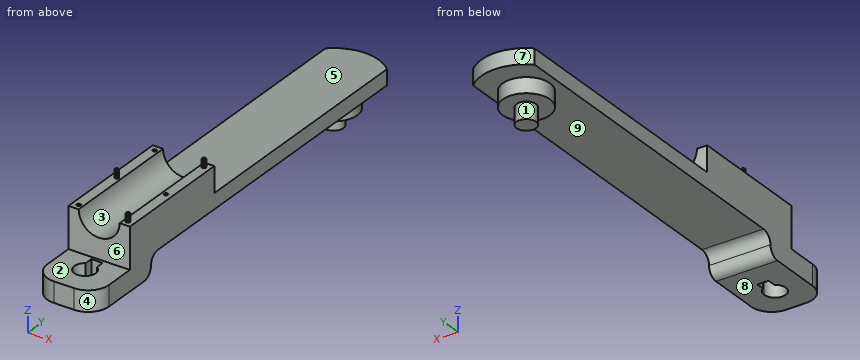
```python
from build123d import *

# Parameters (mm, degrees)
SKETCH2_W                  = 30
SKETCH2_H                  = 30
BOSS_EXTRUDE1_DEPTH        = 60
FILLET1_R                  = 10
SKETCH3_W                  = 40
SKETCH3_H                  = 25
CUT_EXTRUDE1_DEPTH         = 69.738635424
SKETCH6_W                  = 30
SKETCH6_H                  = 40
BOSS_EXTRUDE2_DEPTH        = 125
SKETCH7_W                  = 30
SKETCH7_H                  = 10
BOSS_EXTRUDE3_DEPTH        = 10
FILLET2_START              = -16
FILLET2_DEPTH              = 32
FILLET2_START_2            = -15
FILLET2_2_DEPTH            = 30
SKETCH8_W                  = 25
SKETCH8_H                  = 70
CUT_EXTRUDE2_DEPTH         = 156.241746963
SKETCH12_W                 = 30
SKETCH12_H                 = 7.5
BOSS_EXTRUDE4_DEPTH        = 65
SKETCH13_W                 = 20
SKETCH13_H                 = 54
CUT_EXTRUDE6_DEPTH         = 6
SKETCH20_R                 = 4.75
AXIS_BASE_DEPTH            = 49.6
CUT_EXTRUDE8_DEPTH         = 212.541958013
CUT_EXTRUDE8_DEPTH_BACK    = 212.541958013
SKETCH19_R                 = 2.5
SKETCH19_W                 = 20
SKETCH19_H                 = 42
CUT_EXTRUDE7_DEPTH         = 26.5
MAKE_HALF_DEPTH            = 225.175347112
ONE_MALE_JACK_DEPTH        = 4
CHAMFER1_SIZE              = 0.2
LPATTERN1_COUNT            = 2
LPATTERN1_PITCH            = 24
LPATTERN1_COUNT_DIR2       = 3
LPATTERN1_PITCH_DIR2       = 27
CHAMFER1_OF_LPATTERN1_SIZE = 0.2
ONE_FEMALE_JACK_DEPTH      = 5
FEMALE_JACKS_COUNT         = 2
FEMALE_JACKS_PITCH         = 24
FEMALE_JACKS_COUNT_DIR2    = 3
FEMALE_JACKS_PITCH_DIR2    = 27
SKETCH26_R                 = 10
MAKE_LIGHER_DEPTH          = 60
SKETCH27_R                 = 11.517379081
BOSS_EXTRUDE5_DEPTH        = 7.45


with BuildPart() as part:
    # Sketch2 → Boss-Extrude1 (new body)
    with BuildSketch(Plane.XY):
        Rectangle(SKETCH2_W, SKETCH2_H)
        with BuildLine():
            ThreePointArc((5.25, 0), (-2.561737691, -4.582575695), (-2.75, 4.472135955))
            Line((-2.75, 4.472135955), (-2.75, 8.5))
            Line((-2.75, 8.5), (0, 8.5))
            Line((0, 8.5), (2.75, 8.5))
            Line((2.75, 8.5), (2.75, 4.472135955))
            ThreePointArc((2.75, 4.472135955), (4.582575695, 2.561737691), (5.25, 0))
        make_face(mode=Mode.SUBTRACT)
    extrude(amount=BOSS_EXTRUDE1_DEPTH)

    # Fillet1
    fillet1_edges = [part.edges().sort_by_distance(p)[0] for p in [
        (15, -15, 30),
        (-15, -15, 30),
    ]]
    fillet(fillet1_edges, radius=FILLET1_R)

    # Sketch3 → Cut-Extrude1 (cut, through all)
    with BuildSketch(Plane.ZY.offset(15)):
        with Locations((30, -2.5)):
            Rectangle(SKETCH3_W, SKETCH3_H)
    extrude(amount=-CUT_EXTRUDE1_DEPTH, mode=Mode.SUBTRACT)

    # Sketch6 → Boss-Extrude2 (add)
    with BuildSketch(Plane(origin=(0, 15, 0), x_dir=(1, 0, 0), z_dir=(0, 1, 0))):
        with Locations((0, -30)):
            Rectangle(SKETCH6_W, SKETCH6_H)
    extrude(amount=BOSS_EXTRUDE2_DEPTH)

    # Sketch7 → Boss-Extrude3 (add)
    with BuildSketch(Plane(origin=(0, 15, 0), x_dir=(1, 0, 0), z_dir=(0, 1, 0))):
        with Locations((0, -5)):
            Rectangle(SKETCH7_W, SKETCH7_H)
        with Locations((0, -55)):
            Rectangle(SKETCH7_W, SKETCH7_H)
    extrude(amount=BOSS_EXTRUDE3_DEPTH)

    # Fillet2: read off the stored shape, not the designer's step
    # Fillet2 outline → Fillet2 (cut)
    with BuildSketch(Plane.YZ.offset(FILLET2_START)):
        with BuildLine():
            ThreePointArc((25, 5), (23.535533906, 1.464466094), (20, 0))
            Line((20, 0), (25, 0))
            Line((25, 0), (25, 5))
        make_face()
        with BuildLine():
            Line((25, 60), (20, 60))
            ThreePointArc((20, 60), (23.535533906, 58.535533906), (25, 55))
            Line((25, 55), (25, 60))
        make_face()
    extrude(amount=FILLET2_DEPTH, mode=Mode.SUBTRACT)

    # Fillet2 2 outline → Fillet2 2 (add)
    with BuildSketch(Plane.YZ.offset(FILLET2_START_2)):
        with BuildLine():
            Line((25, 10), (25, 5))
            ThreePointArc((25, 5), (26.464466094, 8.535533906), (30, 10))
            Line((30, 10), (25, 10))
        make_face()
        with BuildLine():
            ThreePointArc((30, 50), (26.464466094, 51.464466094), (25, 55))
            Line((25, 55), (25, 50))
            Line((25, 50), (30, 50))
        make_face()
    extrude(amount=FILLET2_2_DEPTH)

    # Sketch8 → Cut-Extrude2 (cut, through all)
    with BuildSketch(Plane(origin=(15, 0, 0), x_dir=(0, 0, -1), z_dir=(1, 0, 0))):
        with Locations((-30, 105)):
            Rectangle(SKETCH8_W, SKETCH8_H)
    extrude(amount=-CUT_EXTRUDE2_DEPTH, mode=Mode.SUBTRACT)

    # Sketch12 → Boss-Extrude4 (add)
    with BuildSketch(Plane(origin=(0, 140, 0), x_dir=(1, 0, 0), z_dir=(0, 1, 0))):
        with Locations((0, -13.75)):
            Rectangle(SKETCH12_W, SKETCH12_H)
        with Locations((0, -46.25)):
            Rectangle(SKETCH12_W, SKETCH12_H)
    extrude(amount=BOSS_EXTRUDE4_DEPTH)

    # Sketch13 → Cut-Extrude6 (cut)
    with BuildSketch(Plane.XY.offset(50)):
        with Locations((0, 168)):
            Rectangle(SKETCH13_W, SKETCH13_H)
    extrude(amount=-CUT_EXTRUDE6_DEPTH, mode=Mode.SUBTRACT)

    # Sketch20 → Axis Base (add)
    with BuildSketch(Plane.XY.offset(44)):
        with Locations(Location((0, 176.7, 0), (0, 0, 90))):
            Circle(SKETCH20_R)
    extrude(amount=-AXIS_BASE_DEPTH)

    # Sketch23 → Cut-Extrude8 (cut, two sides: drawn at the far end of the back side and taken through both)
    with BuildSketch(Plane(origin=(0, 0, 10), x_dir=(-1, 0, 0), z_dir=(0, 0, -1)).offset(-CUT_EXTRUDE8_DEPTH_BACK)):
        with BuildLine():
            Line((-15, 192.793476939), (-15, 205))
            Line((-15, 205), (15, 205))
            Line((15, 205), (15, 192.793476939))
            ThreePointArc((15, 192.793476939), (0, 198.7), (-15, 192.793476939))
        make_face()
    extrude(amount=CUT_EXTRUDE8_DEPTH + CUT_EXTRUDE8_DEPTH_BACK, mode=Mode.SUBTRACT)

    # Sketch19 → Cut-Extrude7 (cut)
    with BuildSketch(Plane.XY.offset(44)):
        with Locations((-5.12, 192)):
            Circle(SKETCH19_R)
        with Locations(Location((5.12, 192, 0), (0, 0, 270))):
            Circle(SKETCH19_R)
        with Locations((5.12, 144)):
            Circle(SKETCH19_R)
        with Locations(Location((-5.12, 144, 0), (0, 0, 270))):
            Circle(SKETCH19_R)
        with Locations((0, 168)):
            Rectangle(SKETCH19_W, SKETCH19_H)
    extrude(amount=-CUT_EXTRUDE7_DEPTH, mode=Mode.SUBTRACT)

    # 3DSketch2 → Make Half (cut, through all)
    with BuildSketch(Plane(origin=(-16.97773478, -20.308334844, 30), x_dir=(0.14055892995616934, 0.9900723141314359, 0), z_dir=(0, 0, 1))):
        Polygon((0, 0), (4.55547701, -32.087976668), (230.577525736, 0), (226.022048726, 32.087976668), align=None)
    extrude(amount=MAKE_HALF_DEPTH, mode=Mode.SUBTRACT)

    # Sketch24 → One Male Jack (add)
    with BuildSketch(Plane.XY.offset(30)):
        Polygon((12, 68), (11.292893219, 67.707106781), (11, 67), (11.292893219, 66.292893219), (12, 66), (12.707106781, 66.292893219), (13, 67), (12.707106781, 67.707106781), align=None)
    one_male_jack = extrude(amount=ONE_MALE_JACK_DEPTH)

    # Chamfer1
    chamfer1_edges = [part.edges().sort_by_distance(p)[0] for p in [
        (12.353553391, 67.853553391, 34),
        (11.646446609, 67.853553391, 34),
        (11.146446609, 67.353553391, 34),
        (11.146446609, 66.646446609, 34),
        (11.646446609, 66.146446609, 34),
        (12.353553391, 66.146446609, 34),
        (12.853553391, 66.646446609, 34),
        (12.853553391, 67.353553391, 34),
    ]]
    chamfer(chamfer1_edges, length=CHAMFER1_SIZE)

    # LPattern1: One Male Jack 2 × 3, 3 skipped
    with Locations(*[(-i * LPATTERN1_PITCH, -j * LPATTERN1_PITCH_DIR2, 0) for i in range(LPATTERN1_COUNT) for j in range(LPATTERN1_COUNT_DIR2) if (i, j) not in ((0, 0), (0, 1), (1, 0), (1, 2))]):
        add(one_male_jack)

    # Chamfer1 of LPattern1
    chamfer1_of_lpattern1_edges = [part.edges().sort_by_distance(p)[0] for p in [
        (12.353553391, 13.853553391, 34),
        (11.646446609, 13.853553391, 34),
        (11.146446609, 13.353553391, 34),
        (11.146446609, 12.646446609, 34),
        (11.646446609, 12.146446609, 34),
        (12.353553391, 12.146446609, 34),
        (12.853553391, 12.646446609, 34),
        (12.853553391, 13.353553391, 34),
        (-11.646446609, 40.853553391, 34),
        (-12.353553391, 40.853553391, 34),
        (-12.853553391, 40.353553391, 34),
        (-12.853553391, 39.646446609, 34),
        (-12.353553391, 39.146446609, 34),
        (-11.646446609, 39.146446609, 34),
        (-11.146446609, 39.646446609, 34),
        (-11.146446609, 40.353553391, 34),
    ]]
    chamfer(chamfer1_of_lpattern1_edges, length=CHAMFER1_OF_LPATTERN1_SIZE)

    # Sketch25 → One Female Jack (cut)
    with BuildSketch(Plane.XY.offset(30)):
        Polygon((-12, 68.025), (-12.724784451, 67.724784451), (-13.025, 67), (-12.724784451, 66.275215549), (-12, 65.975), (-11.275215549, 66.275215549), (-10.975, 67), (-11.275215549, 67.724784451), align=None)
    one_female_jack = extrude(amount=-ONE_FEMALE_JACK_DEPTH, mode=Mode.SUBTRACT)

    # Female Jacks: One Female Jack 2 × 3, 3 skipped
    with Locations(*[(i * FEMALE_JACKS_PITCH, -j * FEMALE_JACKS_PITCH_DIR2, 0) for i in range(FEMALE_JACKS_COUNT) for j in range(FEMALE_JACKS_COUNT_DIR2) if (i, j) not in ((0, 0), (0, 1), (1, 0), (1, 2))]):
        add(one_female_jack, mode=Mode.SUBTRACT)

    # Sketch26 → Make Ligher (cut)
    with BuildSketch(Plane.XZ.offset(-10)):
        with Locations((0, 30)):
            Circle(SKETCH26_R)
    extrude(amount=-MAKE_LIGHER_DEPTH, mode=Mode.SUBTRACT)

    # Sketch27 → Boss-Extrude5 (add)
    with BuildSketch(Plane(origin=(0, 0, 10), x_dir=(-1, 0, 0), z_dir=(0, 0, -1))):
        with Locations(Location((0, 176.7, 0), (0, 0, 180))):
            Circle(SKETCH27_R)
    extrude(amount=BOSS_EXTRUDE5_DEPTH)


solid = part.part
```
The listing builds one solid part. Answer for the finished solid, in the listing's coordinates (mm). Face numbers are marked on the shaded views. A direction names the side the tool comes from. Give positions to 0.01 mm unless a question says otherwise; leave off trailing zeros. Order: outer loops, then holes, each group sorted by start corner. A loop starts at its lowest first (then second) coordinate and runs counter-clockwise, first axis right, second up. Notation, with made-up numbers: (-14, 21) -> (4, 21) arc R15 cw to (4, 50) -> close; hole circle Ø7 at (10.25, 87). An arc over 180 degrees is marked (long way). Answer as a JSON object with one key per item and string values. Group by question number.
Item 1: The part is cut by section A-A on x = 0. Write down the section's boundary in (y, z).
Item 2: The part is cut by section D-D on y = 48.5. Write down the section's boundary in (x, z), and give its area (3 significant figures).
Item 3: Determine the mould class of the marked faces 6, 7, 8 and 9 for opening direction Y: pulls with the +Y half, pulls with the -Y half, needs draft (parallel to the pull), parting line crosses it, or undercut.
Item 4: The part is cut by section B-B on y = 176.7. Write down the section's boundary in (x, z).
Item 5: The part is cut by section C-C on z = 7. Write down the section's boundary in (x, y), and give its area (3 significant figures).
Item 6: A tool of negligible diameter and unlimited length cuts with its end or side. For the marked faces 1, 2, 3, 4 and 5, from which of +Z, -Z, +X, -X, +Y, -Y can it reach the whole face along a straight path? Write none if from no direction.
Item 7: Flat-ended cylindrical pins translate along their axes: pin 1 (6 mm diameter, centred on x = 6, z = 23.5, fed in from -Y); pin 2 (7 mm diameter, centred on x = 0, y = 181.5, fed in from -Z); pin 3 (4 mm diameter, centred on x = 11.5, y = 46, fed in from +Z); pin 4 (10 mm diameter, centred on x = -12, y = 144, fed in from +Z). Find the tip coordinate at first contact, or state that the pin passes through.
Item 8: Consider L1, parallel to Y at x = 0, z = 4.5; L2, parallel to Y at x = 3, z = 7.5; L3, parallel to X at y = 0, z = 5. Determine where each line is inside the solid, lowest interval first. Write a range as from..to.
Result set:
{
 "1": {"outline": "(-15, 0) -> (-5.25, 0) -> (-5.25, 10) -> (-15, 10) -> close; (8.5, 0) -> (20, 0) arc R5 ccw to (25, 5) arc R5 cw to (30, 10) -> (165.18, 10) -> (165.18, 2.55) -> (171.95, 2.55) -> (171.95, -5.6) -> (181.45, -5.6) -> (181.45, 2.55) -> (188.22, 2.55) -> (188.22, 10) -> (198.7, 10) -> (198.7, 17.5) -> (70, 17.5) -> (70, 20) -> (10, 20) -> (10, 10) -> (8.5, 10) -> close"},
 "2": {"outline": "(-15, 10) -> (15, 10) -> (15, 30) -> (10, 30) arc R10 cw to (-10, 30) -> (-15, 30) -> close", "area": "443 mm²"},
 "3": {"face 6": "pulls with the -Y half", "face 7": "pulls with the +Y half", "face 8": "needs draft", "face 9": "undercut"},
 "4": {"outline": "(-15, 10) -> (-11.52, 10) -> (-11.52, 2.55) -> (-4.75, 2.55) -> (-4.75, -5.6) -> (4.75, -5.6) -> (4.75, 2.55) -> (11.52, 2.55) -> (11.52, 10) -> (15, 10) -> (15, 17.5) -> (-15, 17.5) -> close"},
 "5": {"outline": "(-15, -5) arc R10 ccw to (-5, -15) -> (5, -15) arc R10 ccw to (15, -5) -> (15, 25.42) -> (-15, 25.42) -> close; circle Ø23.03 at (0, 176.7); hole (-2.75, 4.47) arc R5.25 ccw (long way) to (2.75, 4.47) -> (2.75, 8.5) -> (-2.75, 8.5) -> close", "area": "1,480 mm²"},
 "6": {"face 1": "-Z", "face 2": "+Z, +X, -X, -Y", "face 3": "+Z, +Y, -Y", "face 4": "+Z, -Z, +X, -Y", "face 5": "+Z, +X, -X, +Y"},
 "7": {"pin 1": "y = 10", "pin 2": "z = -5.6", "pin 3": "z = 30", "pin 4": "z = 17.5"},
 "8": {"L1": "-15..-5.25, 8.5..24.97, 165.18..188.22", "L2": "-15..-4.31, 4.31..25.67, 165.58..187.82", "L3": "-15..-5.25, 5.25..15"}
}
